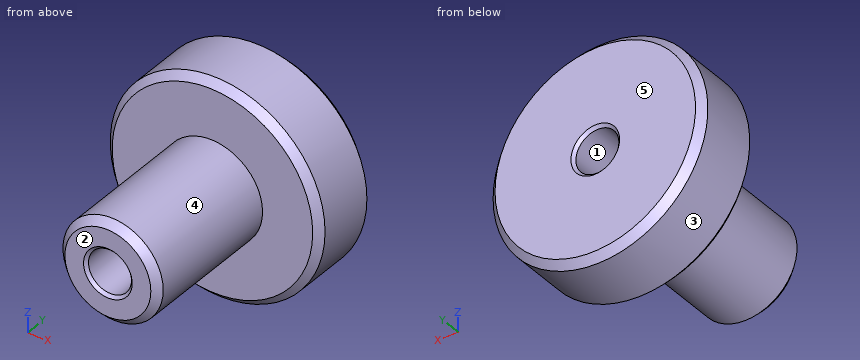
Autodesk Inventor part; units mm, degrees
ref_plane "YZ Plane" through (0, 0, 0) normal (1, 0, 0) x (0, 1, 0)
ref_plane "XZ Plane" through (0, 0, 0) normal (0, 1, 0) x (-1, 0, 0)
ref_plane "XY Plane" through (0, 0, 0) normal (0, 0, 1) x (1, 0, 0)
sketch "Sketch1" plane through (0, 0, 0) normal (0, 0, 1) x (1, 0, 0)
  line L0 (0, 0) -> (0, -15) construction
  line L1 (1.5, 0) -> (7.5, 0)
  line L2 (7.5, 0) -> (7.5, -5)
  line L3 (7.5, -5) -> (3.5, -5)
  line L4 (3.5, -5) -> (3.5, -15)
  line L5 (3.5, -15) -> (1.5, -15)
  line L6 (1.5, -15) -> (1.5, 0)
  dimension "d0" = 1.5
  dimension "d1" = 7.5
  dimension "d2" = 5
  dimension "d3" = 10
  dimension "Length" = 15
  dimension "d5" = 3.5
revolve "Revolution1" add sketch "Sketch1" angle 360 about axis through (0, 0, 0) along (0, -1, 0)
chamfer "Chamfer1" distance 0.5 angle 45 3 edges at (-7.5, 0, 0) (-7.5, -5, 0) (-3.5, -15, 0)
chamfer "Chamfer2" distance 0.2 angle 45 2 edges at (-1.5, 0, 0) (-1.5, -15, 0)
equation "\"Diameter\" = 15"
properties part number "Bush" material "Bronze, Soft Tin"
CAD build for the part. Positions are in the model's coordinates, mm. Face numbers are marked on the shaded views. A direction names the side the tool comes from. Round coordinates to 2 decimals unless told otherwise and drop trailing zeros. Write each loop counter-clockwise with the first axis right and the second up, starting at its lowest first coordinate (ties: lowest second). Pieces come first, ordered by that corner, then holes.
(1) Slice it at B-B, the plane z = 0. Write the cut outline in (x, y).
(2) Slice it at A-A, the plane x = 0. Write the cut outline in (y, z).
(3) 3-axis set-ups, long thin cutter, end or side, ignore diameter. For the marked faces 4 and 5: which of +Z, -Z, +X, -X, +Y, -Y reach the whole face in a straight line?
(4) Slice it at C-C, the plane y = -10.25. Write the cut outline in (x, z), and give its area (3 significant figures).
(5) Mould opens along Z. For the marked faces 1, 2 and 3 say: pulls with the +Z half, pulls with the -Z half, needs draft (parallel to the pull), parting line crosses it, or undercut.
(6) Slice it at D-D, the plane y = -1.75. Write the cut outline in (x, z).
(7) Drop flat-ended pins along their axis: P1, Ø1, axis at y = -7.5, z = 0, coming from the -X side; P2, Ø5, axis at y = -6.5, z = 4, coming from the -X side; P3, Ø1, axis at y = -2, z = 4.5, coming from the -X side. Give the stop position or say it passes through.
(8) Probe line 1 along Z through (x, y) = (0, -9.5); line 2 along Y through (x, z) = (4.75, -4.25); line 3 along X through (y, z) = (-1.75, 0.75). List the from-to ranges inside material, lowest first.
From the geometry:
1. outline: (-7.5, -4.5) - (-7, -5) - (-3.5, -5) - (-3.5, -14.5) - (-3, -15) - (-1.7, -15) - (-1.5, -14.8) - (-1.5, -0.2) - (-1.7, 0) - (-7, 0) - (-7.5, -0.5) - close; (1.5, -14.8) - (1.7, -15) - (3, -15) - (3.5, -14.5) - (3.5, -5) - (7, -5) - (7.5, -4.5) - (7.5, -0.5) - (7, 0) - (1.7, 0) - (1.5, -0.2) - close
2. outline: (-15, -3) - (-14.5, -3.5) - (-5, -3.5) - (-5, -7) - (-4.5, -7.5) - (-0.5, -7.5) - (0, -7) - (0, -1.7) - (-0.2, -1.5) - (-14.8, -1.5) - (-15, -1.7) - close; (-15, 1.7) - (-14.8, 1.5) - (-0.2, 1.5) - (0, 1.7) - (0, 7) - (-0.5, 7.5) - (-4.5, 7.5) - (-5, 7) - (-5, 3.5) - (-14.5, 3.5) - (-15, 3) - close
3. face 4: -Y
3. face 5: +Z, -Z, +X, -X, +Y
4. outline: circle Ø7 at (0, 0); hole circle Ø3 at (0, 0)
4. area: 31.4 mm2
5. face 1: undercut
5. face 2: needs draft
5. face 3: parting line crosses it
6. outline: circle Ø15 at (0, 0); hole circle Ø3 at (0, 0)
7. P1: stops at x = -3.5
7. P2: stops at x = -7.07
7. P3: stops at x = -6.34
8. line 1: z = -3.5 to -1.5, 1.5 to 3.5
8. line 2: y = -5 to 0
8. line 3: x = -7.46 to -1.3, 1.3 to 7.46
